For this review, use the dimensioned drawing (mm, ordinates from the lowest corner) and the shaded views. Give positions to 0.01 mm unless a question says otherwise; leave off trailing zeros. Order: outer loops, then holes, each group sorted by start corner. A loop starts at its lowest first (then second) coordinate and runs counter-clockwise, first axis right, second up.
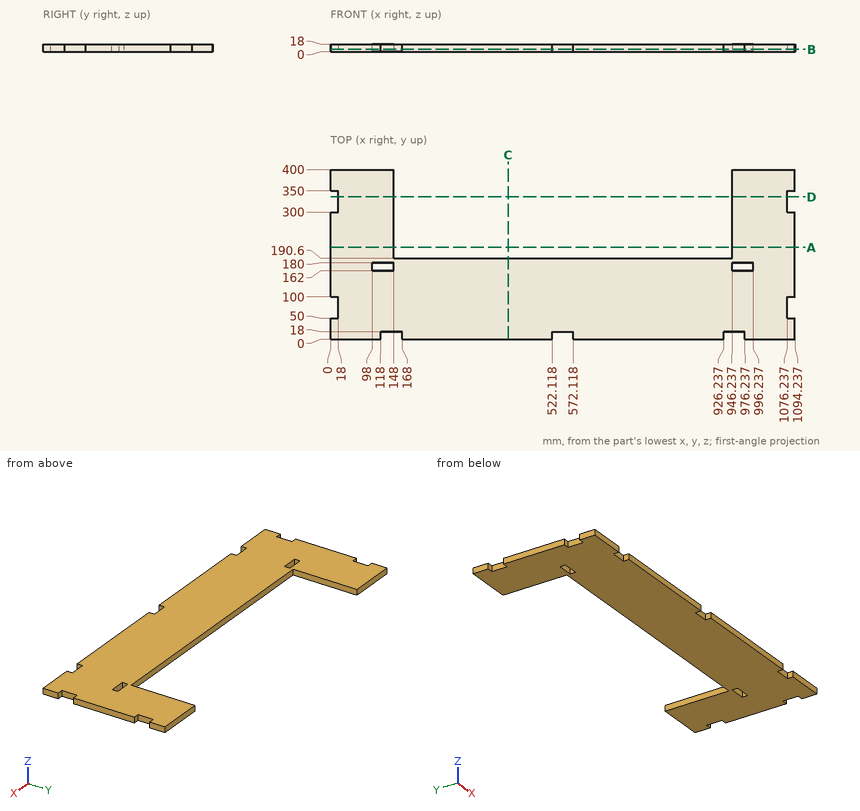
1. For pin 1 (1.5 mm diameter, centred on x = 385, z = 14.5, fed in from +Y); pin 2 (1.5 mm diameter, centred on y = 94, z = 10.5, fed in from -X); pin 3 (5.5 mm diameter, centred on x = 146.5, z = 8.5, fed in from -Y), all flat-tipped, find the tip position at first contact; note any pin that passes through.
Recorded:
pin 1: stops at y = 190.6
pin 2: stops at x = 18
pin 3: stops at y = 18
2. Take a section at C-C (x = 418). State the section outline as (y, z) points.
Recorded:
outline: (0, 0) - (190.6, 0) - (190.6, 18) - (0, 18) - close
3. For line 1 along X through (y, z) = (175, 7.5); line 2 along Y through (x, z) = (959.5, 12.75); line 3 along X through (y, z) = (281.5, 12.75), list the stretches that pass through material, from the lowest coordinate up.
Recorded:
line 1: x = 0 to 98, 148 to 946.24, 996.24 to 1094.24
line 2: y = 18 to 162, 180 to 400
line 3: x = 0 to 148, 946.24 to 1094.24
4. Take a section at D-D (y = 336). State the section outline as (x, z) points, then the cut area to 3 significant figures.
Recorded:
outline: (18, 0) - (148, 0) - (148, 18) - (18, 18) - close; (946.24, 0) - (1076.24, 0) - (1076.24, 18) - (946.24, 18) - close
area: 4,680 mm2
5. Take a section at A-A (y = 216.5). State the section outline as (x, z) points.
Recorded:
outline: (0, 0) - (148, 0) - (148, 18) - (0, 18) - close; (946.24, 0) - (1094.24, 0) - (1094.24, 18) - (946.24, 18) - close
6. Take a section at B-B (z = 5.25). State how many separate pieces and enclosed holes the cut face has, then the cut area to 3 significant figures.
Recorded:
separate pieces: 1
enclosed holes: 2
area: 262,000 mm2
